Geometry: final body of the model. Coordinates: model frame, mm. Give positions to 0.01 mm unless a question says otherwise; leave off trailing zeros. Write each loop counter-clockwise with the first axis right and the second up, starting at its lowest first coordinate (ties: lowest second). Pieces come first, ordered by that corner, then holes. Notation, with made-up numbers: (66, 5) -> (93, 5) arc R10 cw to (93, 11) -> close; hole circle Ø7 at (29.5, 33.25). An arc over 180 degrees is marked (long way). Answer in a Markdown table with one row per item. Add a question column.
Item 1: Section query D-D on x = 436. Output: boundary loops of the cut face in (y, z).
Item 2: First-contact query: P1, Ø2, axis at y = 1.5, z = 204, coming from the -X side; P2, Ø1, axis at x = 364, y = 3, coming from the -Z side; P3, Ø1.2, axis at y = 1.5, z = 205.5, coming from the +X side. Flat tips, straight axial feed; report the tip coordinate or a pass-through.
Item 3: Section query B-B on y = 2.7. State how many separate pieces and enclosed holes the cut face has, plus the area to 3 significant figures.
Item 4: Material intervals for probe 1 along Z at (x, y) = (375.5, 2.5); probe 2 along Z at (x, y) = (371, 1.65); probe 3 along X at (y, z) = (1.8, 271), sorted ascending. Write a range as from..to.
Item 5: Section query C-C on z = 162. Output: boundary loops of the cut face in (x, y).
Item 6: Section query A-A on z = 132.5. Output: boundary loops of the cut face in (x, y), plus the area to 3 significant figures.
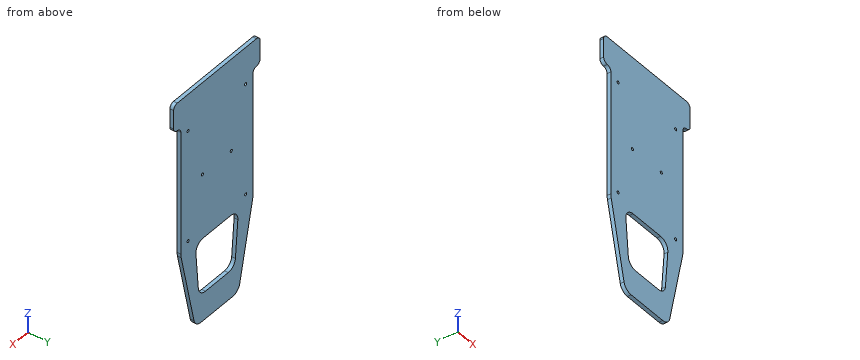
```python
from build123d import *

# Parameters (mm, degrees)
SKETCH_1_R      = 1.5
EXTRUDE_1_DEPTH = 4
FILLET_1_R      = 5
FILLET_2_R      = 20
FILLET_3_R      = 10
FILLET_4_R      = 10


with BuildPart() as part:
    # Эскиз1 → Бобышка-Вытянуть1 (new body)
    with BuildSketch(Plane(origin=(0, 0, 0), x_dir=(1, 0, 0), z_dir=(0, 1, 0))):
        Polygon((341.185276631, -307.117267335), (341.185276631, -167.117267335), (361.185276631, -77.117267335), (421.185276631, -77.117267335), (441.185276631, -167.117267335), (441.185276631, -307.117267335), (451.185276631, -307.117267335), (451.185276631, -337.117267335), (391.185276631, -337.117267335), (331.185276631, -337.117267335), (331.185276631, -307.117267335), align=None)
        with Locations(Location((351.185276631, -177.117267335, 0), (0, 0, 270))):
            Circle(SKETCH_1_R, mode=Mode.SUBTRACT)
        with Locations(Location((431.185276631, -177.117267335, 0), (0, 0, 270))):
            Circle(SKETCH_1_R, mode=Mode.SUBTRACT)
        with Locations(Location((431.185276631, -297.117267335, 0), (0, 0, 270))):
            Circle(SKETCH_1_R, mode=Mode.SUBTRACT)
        with Locations(Location((351.185276631, -297.117267335, 0), (0, 0, 270))):
            Circle(SKETCH_1_R, mode=Mode.SUBTRACT)
        with Locations(Location((371.185276631, -237.117267335, 0), (0, 0, 270))):
            Circle(SKETCH_1_R, mode=Mode.SUBTRACT)
        with Locations(Location((411.185276631, -237.117267335, 0), (0, 0, 270))):
            Circle(SKETCH_1_R, mode=Mode.SUBTRACT)
        Polygon((361.185276631, -167.117267335), (366.185276631, -107.117267335), (416.185276631, -107.117267335), (421.185276631, -167.117267335), align=None, mode=Mode.SUBTRACT)
    extrude(amount=EXTRUDE_1_DEPTH)

    # Скругление1
    fillet_1_edges = [part.edges().sort_by_distance(p)[0] for p in [
        (441.185276631, 2, 307.117267335),
        (341.185276631, 2, 307.117267335),
        (331.185276631, 2, 307.117267335),
        (331.185276631, 2, 337.117267335),
        (451.185276631, 2, 337.117267335),
        (451.185276631, 2, 307.117267335),
    ]]
    fillet(fillet_1_edges, radius=FILLET_1_R - 0.0001)  # a hair under: the kernel refuses the full size

    # Скругление2
    fillet_2_edges = [part.edges().sort_by_distance(p)[0] for p in [
        (441.185276631, 2, 167.117267335),
        (341.185276631, 2, 167.117267335),
    ]]
    fillet(fillet_2_edges, radius=FILLET_2_R)

    # Скругление3
    fillet_3_edges = [part.edges().sort_by_distance(p)[0] for p in [
        (416.185276631, 2, 107.117267335),
        (366.185276631, 2, 107.117267335),
        (361.185276631, 2, 167.117267335),
        (421.185276631, 2, 167.117267335),
    ]]
    fillet(fillet_3_edges, radius=FILLET_3_R)

    # Скругление4
    fillet_4_edges = [part.edges().sort_by_distance(p)[0] for p in [
        (361.185276631, 2, 77.117267335),
        (421.185276631, 2, 77.117267335),
    ]]
    fillet(fillet_4_edges, radius=FILLET_4_R)


solid = part.part
```
Findings below:
| question | item | result |
|---|---|---|
| 1 | outline | (0, 143.78) -> (4, 143.78) -> (4, 337.12) -> (0, 337.12) -> close |
| 2 | P1 | stops at x = 341.19 |
| 2 | P2 | stops at z = 78.29 |
| 2 | P3 | stops at x = 441.19 |
| 3 | separate pieces | 1 |
| 3 | enclosed holes | 7 |
| 3 | area | 21,500 mm^2 |
| 4 | probe 1 | z = 77.12..107.12, 167.12..337.12 |
| 4 | probe 2 | z = 77.12..108.13, 167.06..235.63, 238.61..337.12 |
| 4 | probe 3 | x = 341.19..441.19 |
| 5 | outline | (342.32, 0) -> (363.33, 0) -> (363.33, 4) -> (342.32, 4) -> close; (419.04, 0) -> (440.05, 0) -> (440.05, 4) -> (419.04, 4) -> close |
| 6 | outline | (348.88, 0) -> (364.07, 0) -> (364.07, 4) -> (348.88, 4) -> close; (418.3, 0) -> (433.49, 0) -> (433.49, 4) -> (418.3, 4) -> close |
| 6 | area | 122 mm^2 |
